Source: CAD feature listing. Evaluate the final solid. Frame: model axes, mm. Face numbers are marked on the shaded views. A direction names the side the tool comes from. Round coordinates to 2 decimals unless told otherwise and drop trailing zeros. Write each loop counter-clockwise with the first axis right and the second up, starting at its lowest first coordinate (ties: lowest second). Pieces come first, ordered by that corner, then holes. Notation, with made-up numbers: M 34.25,57.5 L 83.25,57.5 A28 cw 83.25,89.5 Z; hole C -2,-6.75 d4. An arc over 180 degrees is marked long. Use a Markdown table: item, result.
```python
from build123d import *

# Parameters (mm, degrees)
BOSS_EXTRUDE1_DEPTH = 3.2
SKETCH2_W           = 40
SKETCH2_H           = 27.451745852
BOSS_EXTRUDE2_DEPTH = 2


with BuildPart() as part:
    # Sketch1 → Boss-Extrude1 (new body)
    with BuildSketch(Plane(origin=(0, 0, 0), x_dir=(1, 0, 0), z_dir=(0, 1, 0))):
        Polygon((10.5, -10.873040155), (10.5, -13.725872926), (20, -13.725872926), (20, 13.725872926), (-20, 13.725872926), (-20, -13.725872926), (0.5, -13.725872926), (0.5, -10.873040155), (-11.5, -10.873040155), (-11.5, -6.873040155), (-16, -6.873040155), (-16, -4.873040155), (-11.5, -4.873040155), (-11.5, 10.626959845), (11.5, 10.626959845), (11.5, -4.873040155), (16, -4.873040155), (16, -6.873040155), (11.5, -6.873040155), (11.5, -10.873040155), align=None)
    extrude(amount=BOSS_EXTRUDE1_DEPTH)

    # Sketch2 → Boss-Extrude2 (add)
    with BuildSketch(Plane(origin=(0, 3.2, 0), x_dir=(1, 0, 0), z_dir=(0, 1, 0))):
        Rectangle(SKETCH2_W, SKETCH2_H)
    extrude(amount=BOSS_EXTRUDE2_DEPTH)


solid = part.part
```
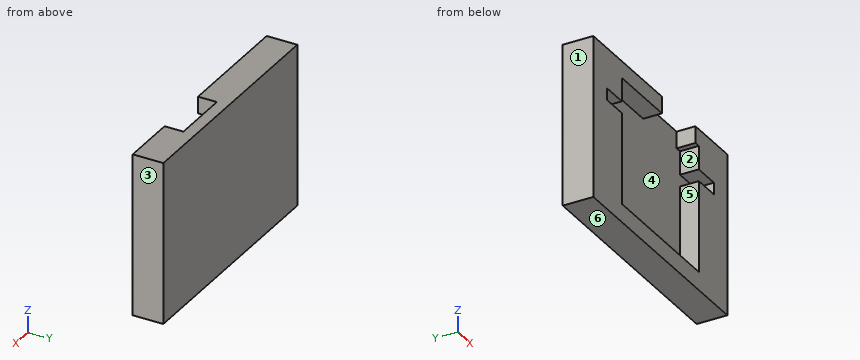
Q1. Section B-B on x = 9. Return loops of the section in (y, z), plus the area to 3 significant figures.
Results are:
| item | result |
|---|---|
| outline | M 0,-13.73 L 5.2,-13.73 L 5.2,13.73 L 3.2,13.73 L 3.2,-10.63 L 0,-10.63 Z |
| area | 64.8 mm^2 |
Q2. Section A-A on z = 6. Return loops of the section in (x, y), plus the area to 3 significant figures.
Results are:
| item | result |
|---|---|
| outline | M -20,0 L -16,0 L -16,3.2 L 16,3.2 L 16,0 L 20,0 L 20,5.2 L -20,5.2 Z |
| area | 106 mm^2 |
Q3. Mould query, pull axis Z, two halves, no side actions, for the marked faces 3, 4, 5 and 6. Classes: +Z half, -Z half, draft (parallel to the pull), parting line (faces both ways), or undercut.
Results are:
| item | result |
|---|---|
| face 3 | draft |
| face 4 | undercut |
| face 5 | undercut |
| face 6 | -Z half |
Q4. Reachability of the marked faces 1 and 2 from +Z, -Z, +X, -X, +Y, -Y: full face, straight path, thin tool, end or side. Return the list, or none.
Results are:
| item | result |
|---|---|
| face 1 | +Z, -Z, -X, +Y, -Y |
| face 2 | -Y |
Q5. Section D-D on x = -15.5. Return loops of the section in (y, z).
Results are:
| item | result |
|---|---|
| outline | M 0,-13.73 L 5.2,-13.73 L 5.2,13.73 L 0,13.73 L 0,6.87 L 3.2,6.87 L 3.2,4.87 L 0,4.87 Z |
Q6. Section C-C on y = 2.1. Return loops of the section in (x, z), plus the area to 3 significant figures.
Results are:
| item | result |
|---|---|
| outline | M -20,-13.73 L 20,-13.73 L 20,13.73 L 10.5,13.73 L 10.5,10.87 L 11.5,10.87 L 11.5,6.87 L 16,6.87 L 16,4.87 L 11.5,4.87 L 11.5,-10.63 L -11.5,-10.63 L -11.5,4.87 L -16,4.87 L -16,6.87 L -11.5,6.87 L -11.5,10.87 L 0.5,10.87 L 0.5,13.73 L -20,13.73 Z |
| area | 557 mm^2 |
Q7. Line query: L1, parallel to X at y = 2.4, z = 9.5; L2, parallel to Z at x = -3, y = 1.75; L3, parallel to Y at x = 2.5, z = 6.75. Output: solid intervals per line, ascending.
Results are:
| item | result |
|---|---|
| L1 | -20 to -11.5, 11.5 to 20 |
| L2 | -13.73 to -10.63, 10.87 to 13.73 |
| L3 | 3.2 to 5.2 |
